```python
from build123d import *

# Parameters (mm, degrees)
SKETCH_1_R           = 14
EXTRUDE_1_DEPTH      = 22
SKETCH_3_R           = 7.35
CUT_EXTRUDE_1_DEPTH  = 6
SKETCH_2_R           = 1.1
CUT_EXTRUDE_2_DEPTH  = 32
SKETCH_4_R           = 1.85
CUT_EXTRUDE_3_DEPTH  = 17
SKETCH_5_W           = 5.15
SKETCH_5_H           = 5.15
CUT_EXTRUDE_4_DEPTH  = 13
EXTRUDE_2_REACH      = 32.899
CUT_EXTRUDE_7_DEPTH  = 20
SKETCH_11_R          = 4.05
CUT_EXTRUDE_8_DEPTH  = 2
SKETCH_12_R          = 19.208398283
CUT_EXTRUDE_9_DEPTH  = 4
SKETCH_13_R          = 1.5
CUT_EXTRUDE_10_DEPTH = 23
FILLET_1_R           = 2


with BuildPart() as part:
    # 草图1 → 凸台-拉伸1 (new body)
    with BuildSketch(Plane.XY):
        Circle(SKETCH_1_R)
    extrude(amount=EXTRUDE_1_DEPTH)

    # 草图3 → 切除-拉伸1 (cut)
    with BuildSketch(Plane(origin=(0, 0, 0), x_dir=(-1, 0, 0), z_dir=(0, 0, -1))):
        Circle(SKETCH_3_R)
    extrude(amount=-CUT_EXTRUDE_1_DEPTH, mode=Mode.SUBTRACT)

    # 草图2 → 切除-拉伸2 (cut)
    with BuildSketch(Plane.XY.offset(22)):
        with Locations((-9.09326674, -5.25)):
            Circle(SKETCH_2_R)
        with Locations((-9.09326674, 5.25)):
            Circle(SKETCH_2_R)
        with Locations((0, 10.5)):
            Circle(SKETCH_2_R)
        with Locations((9.09326674, 5.25)):
            Circle(SKETCH_2_R)
        with Locations((9.09326674, -5.25)):
            Circle(SKETCH_2_R)
        with Locations((0, -10.5)):
            Circle(SKETCH_2_R)
    extrude(amount=-CUT_EXTRUDE_2_DEPTH, mode=Mode.SUBTRACT)

    # 草图4 → 切除-拉伸3 (cut)
    with BuildSketch(Plane.XY.offset(22)):
        with Locations((9.09326674, 5.25)):
            Circle(SKETCH_4_R)
        with Locations((9.09326674, -5.25)):
            Circle(SKETCH_4_R)
        with Locations((0, -10.5)):
            Circle(SKETCH_4_R)
        with Locations((-9.09326674, -5.25)):
            Circle(SKETCH_4_R)
        with Locations((-9.09326674, 5.25)):
            Circle(SKETCH_4_R)
        with Locations((0, 10.5)):
            Circle(SKETCH_4_R)
    extrude(amount=-CUT_EXTRUDE_3_DEPTH, mode=Mode.SUBTRACT)

    # 草图5 → 切除-拉伸4 (cut)
    with BuildSketch(Plane.XY.offset(22)):
        Rectangle(SKETCH_5_W, SKETCH_5_H)
    extrude(amount=-CUT_EXTRUDE_4_DEPTH, mode=Mode.SUBTRACT)

    # 草图6 → 凸台-拉伸2 (add, up to next)
    with BuildSketch(Plane(origin=(-2.575, 0, 0), x_dir=(0, 0, -1), z_dir=(1, 0, 0)), mode=Mode.PRIVATE) as extrude_2_sk1:
        Polygon((-9, -2.575), (-14.15, -2.575), (-9, 2.575), align=None)
    extrude_2_tool1 = extrude(extrude_2_sk1.sketch, amount=EXTRUDE_2_REACH, mode=Mode.PRIVATE) - part.part
    add(extrude_2_tool1.solids().sort_by_distance((-2.575, -0.858333, 10.716667))[0])

    # 草图9 → 切除-拉伸7 (cut)
    with BuildSketch(Plane(origin=(0, 2.575, 0), x_dir=(-1, 0, 0), z_dir=(0, -1, 0))):
        with BuildLine():
            Line((2, -11), (2, -13))
            ThreePointArc((2, -13), (0, -15), (-2, -13))
            Line((-2, -13), (-2, -11))
            ThreePointArc((-2, -11), (0, -9), (2, -11))
        make_face()
    extrude(amount=-CUT_EXTRUDE_7_DEPTH, mode=Mode.SUBTRACT)

    # 草图11 → 切除-拉伸8 (cut, symmetric)
    with BuildSketch(Plane(origin=(0, 13.416407865, 0), x_dir=(1, 0, 0), z_dir=(0, 1, 0))):
        with Locations(Location((0, -11, 0), (0, 0, 90))):
            Circle(SKETCH_11_R)
    extrude(amount=CUT_EXTRUDE_8_DEPTH, both=True, mode=Mode.SUBTRACT)

    # 草图12 → 切除-拉伸9 (cut)
    with BuildSketch(Plane.XY.offset(22)):
        Circle(SKETCH_12_R)
    extrude(amount=-CUT_EXTRUDE_9_DEPTH, mode=Mode.SUBTRACT)

    # 草图13 → 切除-拉伸10 (cut)
    with BuildSketch(Plane(origin=(0, 2.575, 0), x_dir=(-1, 0, 0), z_dir=(0, -1, 0))):
        with Locations(Location((0, -11, 0), (0, 0, 270))):
            Circle(SKETCH_13_R)
    extrude(amount=CUT_EXTRUDE_10_DEPTH, mode=Mode.SUBTRACT)

    # 圆角1
    # the kernel refuses this fillet: 2 mm, written as the material it takes off along each edge
    with BuildSketch(Plane(origin=(0, 0, 18), x_dir=(1, 0, 0), z_dir=(0, 1, 0))) as fillet_1_piece_1:
        with BuildLine():
            CenterArc((14 - FILLET_1_R, FILLET_1_R), FILLET_1_R, 270, 90)
            Line((14, FILLET_1_R), (14, 0))
            Line((14, 0), (14 - FILLET_1_R, 0))
        make_face()
    revolve(axis=Axis((0, 0, 18), (0, 0, -1)), mode=Mode.SUBTRACT)


solid = part.part
```
Input: part model. Units: mm. Frame: model coordinates. A direction names the side the tool comes from. Coordinates: 2 decimals unless noted, no trailing zeros. Order: outer loops, then holes, each group sorted by start corner. A loop starts at its lowest first (then second) coordinate and runs counter-clockwise, first axis right, second up. Notation, with made-up numbers: (89.5, 34) - (138.5, 34) arc R31 cw to (138.5, 67) - close; hole circle Ø6 at (1.5, 17). An arc over 180 degrees is marked (long way). Put each result on its own line as item: value.
1. Cut plane B-B on z = 3.5. Return the cut outline in (x, y), then the cut area to 3 significant figures.
Report:
outline: circle Ø28 at (0, 0); hole circle Ø2.2 at (-9.09, -5.25); hole circle Ø2.2 at (-9.09, 5.25); hole circle Ø14.7 at (0, 0); hole circle Ø2.2 at (0, -10.5); hole circle Ø2.2 at (0, 10.5); hole circle Ø2.2 at (9.09, -5.25); hole circle Ø2.2 at (9.09, 5.25)
area: 423 mm2
2. Draft query along Y for faces 1 (the face through (6.5, -12.4, 7.9)), 2 (the face through (0, -2.575, 16)), 3 (the face through (7.73, -4, 11.59)), 4 (the face through (2, 7, 12)). Return one class per face: pulls with the +Y half, pulls with the -Y half, needs draft (parallel to the pull), parting line crosses it, or undercut.
Report:
face 1: parting line crosses it
face 2: undercut
face 3: undercut
face 4: needs draft
3. Cut plane C-C on y = 4.5. State how many separate pieces and enclosed holes the cut face has, then the cut area to 3 significant figures.
Report:
separate pieces: 3
enclosed holes: 1
area: 281 mm2
4. Cut plane A-A on z = 15.5. Return the cut outline in (x, y) (3 decimals).
Report:
outline: circle Ø28 at (0, 0); hole circle Ø3.7 at (-9.093, -5.25); hole circle Ø3.7 at (-9.093, 5.25); hole (-2.575, -2.575) - (2.575, -2.575) - (2.575, 2.575) - (-2.575, 2.575) - close; hole circle Ø3.7 at (0, -10.5); hole circle Ø3.7 at (0, 10.5); hole circle Ø3.7 at (9.093, -5.25); hole circle Ø3.7 at (9.093, 5.25)
5. Contact query for flat-ended pins moving along their axis: pin 1 Ø3 at (x, y) = (-9.09, 5.25) entering from +Z; pin 2 Ø1.8 at (x, y) = (0, 10.5) entering from -Z; pin 3 Ø1.5 at (y, z) = (1, 14) entering from +X; pin 4 Ø1 at (y, z) = (4, 4) entering from +X. Output: stop coordinate, or through.
Report:
pin 1: stops at z = 5
pin 2: passes through
pin 3: stops at x = 14
pin 4: stops at x = 13.56
6. Cut plane D-D on y = 0. Return the cut outline in (x, z) (3 decimals), then the cut area to 3 significant figures.
Report:
outline: (-14, 0) - (-7.35, 0) - (-7.35, 6) - (7.35, 6) - (7.35, 0) - (14, 0) - (14, 16) arc R2 ccw to (12, 18) - (2.575, 18) - (2.575, 11.575) - (1.385, 11.575) arc R1.5 cw (long way) to (-1.385, 11.575) - (-2.575, 11.575) - (-2.575, 18) - (-12, 18) arc R2 ccw to (-14, 16) - close
area: 376 mm2
7. Line query: line 1 along Y through (x, z) = (0, 2.55); line 2 along X through (y, z) = (-5.25, 13.25); line 3 along X through (y, z) = (6.25, 3.5) (3 decimals). Output: solid intervals per line, ascending.
Report:
line 1: y = -14 to -11.6, -9.4 to -7.35, 7.35 to 9.4, 11.6 to 14
line 2: x = -12.98 to -10.94, -7.24 to 7.24, 10.94 to 12.98
line 3: x = -12.527 to -9.552, -8.635 to -3.868, 3.868 to 8.635, 9.552 to 12.527
8. Reachability of faces 5 (the face through (-8.044, -4.92, 2.535)), 6 (the face through (-1.85, -10.42, 11.59)) from +Z, -Z, +X, -X, +Y, -Y: full face, straight path, thin tool, end or side. Return the list, or none.
Report:
face 5: +Z, -Z
face 6: +Z
